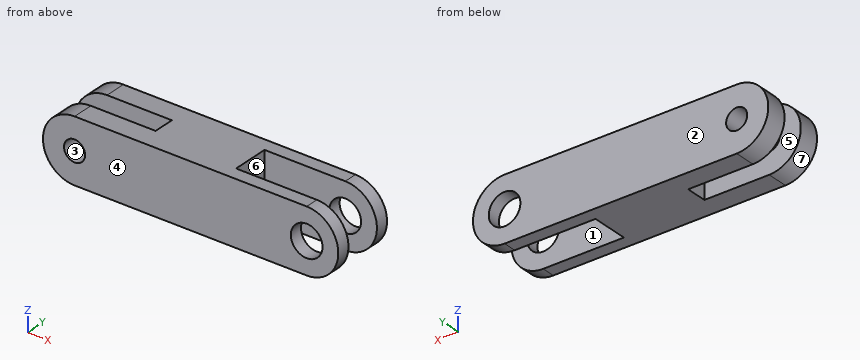
```python
from build123d import *

# Parameters (mm, degrees)
SKETCH_1_R          = 1.5
SKETCH_1_R_2        = 1
EXTRUDE_1_DEPTH     = 3
SKETCH_6_W          = 31.511370345
SKETCH_6_H          = 11.605197544
CUT_EXTRUDE_2_DEPTH = 1.75
SKETCH_7_W          = 12.660216836
SKETCH_7_H          = 9.649927943
CUT_EXTRUDE_3_DEPTH = 1


with BuildPart() as part:
    # 草图1 → 凸台-拉伸1 (new, symmetric)
    with BuildSketch(Plane(origin=(0, 0, 0), x_dir=(1, 0, 0), z_dir=(0, 1, 0))):
        with BuildLine():
            Line((0, 3), (22, 3))
            ThreePointArc((22, 3), (25, 0), (22, -3))
            Line((22, -3), (0, -3))
            ThreePointArc((0, -3), (-3, 0), (0, 3))
        make_face()
        with Locations(Location((22, 0, 0), (0, 0, 270))):
            Circle(SKETCH_1_R, mode=Mode.SUBTRACT)
        with Locations(Location((0, 0, 0), (0, 0, 270))):
            Circle(SKETCH_1_R_2, mode=Mode.SUBTRACT)
    extrude(amount=EXTRUDE_1_DEPTH, both=True)

    # 草图6 → 切除-拉伸2 (cut, symmetric)
    with BuildSketch(Plane(origin=(0, 0, 0), x_dir=(1, 0, 0), z_dir=(0, 1, 0))):
        with Locations((30.101826092, 2.040608699)):
            Rectangle(SKETCH_6_W, SKETCH_6_H)
    extrude(amount=CUT_EXTRUDE_2_DEPTH, both=True, mode=Mode.SUBTRACT)

    # 草图7 → 切除-拉伸3 (cut, symmetric)
    with BuildSketch(Plane(origin=(0, 0, 0), x_dir=(1, 0, 0), z_dir=(0, 1, 0))):
        with Locations((-0.191074288, 0.210879474)):
            Rectangle(SKETCH_7_W, SKETCH_7_H)
    extrude(amount=CUT_EXTRUDE_3_DEPTH, both=True, mode=Mode.SUBTRACT)


solid = part.part
```
The model under review builds one solid part; all positions refer to its coordinate system, in mm. Face numbers are marked on the shaded views. A direction names the side the tool comes from. Round coordinates to 2 decimals unless told otherwise and drop trailing zeros. Loops run counter-clockwise (first coordinate to the right, second up) from the corner with the lowest first, then second, coordinate; pieces in that order, holes last. Notation, with made-up numbers: M 34.5,75 L 78.5,75 A14 ccw 78.5,92 Z; hole C -2.75,54.25 d7. An arc over 180 degrees is marked long. Put each result on its own line as item: value.
Q1. Machinability: for the marked faces 5, 6 and 7, which of the approach directions +Z, -Z, +X, -X, +Y, -Y give a long, thin tool a straight path to every point of the face, cutting with its end or side? Answer none if there is none.
Result set:
face 5: +Z, -Z, -X
face 6: +Z, -Z, +X
face 7: -X, +Y, -Y
Q2. Consider section A-A, the plane x = 17.75. Give the boundary of the cut face in (y, z).
Result set:
outline: M -3,-3 L -1.75,-3 L -1.75,3 L -3,3 Z; M 1.75,-3 L 3,-3 L 3,3 L 1.75,3 Z
Q3. Consider section B-B, the plane z = 0. Give the boundary of the cut face in (x, y), then the cut area to 3 significant figures.
Result set:
outline: M -3,-3 L -1,-3 L -1,-1 L -3,-1 Z; M -3,1 L -1,1 L -1,3 L -3,3 Z; M 1,-3 L 20.5,-3 L 20.5,-1.75 L 14.35,-1.75 L 14.35,1.75 L 20.5,1.75 L 20.5,3 L 1,3 L 1,1 L 6.14,1 L 6.14,-1 L 1,-1 Z; M 23.5,-3 L 25,-3 L 25,-1.75 L 23.5,-1.75 Z; M 23.5,1.75 L 25,1.75 L 25,3 L 23.5,3 Z
area: 96.9 mm²
Q4. Mouldability with a two-part tool opening along Y and no side actions: class the marked faces 1, 2, 3 and 4 as released by +Y, released by -Y, zero draft, split by the parting line, or undercut.
Result set:
face 1: undercut
face 2: released by +Y
face 3: zero draft
face 4: released by -Y
Q5. Consider section D-D, the plane y = 2.3. Give the boundary of the cut face in (x, z), then the cut area to 3 significant figures.
Result set:
outline: M 0,-3 L 22,-3 A3 ccw 22,3 L 0,3 A3 ccw Z; hole C 0,0 d2; hole C 22,0 d3
area: 150 mm²
Q6. For pin 1 (1 mm diameter, centred on y = 0, z = -2, fed in from -X); pin 2 (1.5 mm diameter, centred on y = 0.5, z = 1, fed in from +X); pin 3 (2.5 mm diameter, centred on x = 22, z = 0, fed in from +Y), all flat-tipped, find the tip position at first contact; note any pin that passes through.
Result set:
pin 1: stops at x = 6.14
pin 2: stops at x = 14.35
pin 3: passes through
Q7. Consider section C-C, the plane z = -1.8. Give the boundary of the cut face in (x, y).
Result set:
outline: M -2.4,-3 L 24.4,-3 L 24.4,-1.75 L 14.35,-1.75 L 14.35,1.75 L 24.4,1.75 L 24.4,3 L -2.4,3 L -2.4,1 L 6.14,1 L 6.14,-1 L -2.4,-1 Z
Q8. To check wall thickness, follow L1, parallel to X at y = 1.9, z = 0; L2, parallel to Y at x = 2.75, z = -2.45; L3, parallel to Z at x = 22, y = -2.1. State the ranges of each line that lie inside material, in increasing order.
Result set:
L1: x = -3 to -1, 1 to 20.5, 23.5 to 25
L2: y = -3 to -1, 1 to 3
L3: z = -3 to -1.5, 1.5 to 3
